Work out the finished part from the listing and answer in its coordinate system (mm). A direction names the side the tool comes from. Coordinates: 2 decimals unless noted, no trailing zeros. Order: outer loops, then holes, each group sorted by start corner. A loop starts at its lowest first (then second) coordinate and runs counter-clockwise, first axis right, second up. Notation, with made-up numbers: M -31,47 L 17,47 A30 ccw 17,81 Z; hole C 75,-9.5 d6. An arc over 180 degrees is marked long. Answer in a Markdown table with one row per item. Add a question column.
Item 1: The part is cut by section C-C (x = -29.5). Write down the section's boundary in (y, z), then the cut area to 3 significant figures.
Item 2: Which of the six approach directions +Z, -Z, +X, -X, +Y, -Y give full straight-line access (tool end or side, diameter ignored) to faces 4 (the face through (63.945, -1, 10)), 5 (the face through (39, -26, 2.67))?
Item 3: The mould has two halves that part along Y. Classify faces 1 (the face through (-1, 1, 20.2)), 2 (the face through (13, 0, 2.67)), 3 (the face through (-1, -42.8, 10)): released by +Y, released by -Y, zero draft, split by the parting line, or undercut.
Item 4: The part is cut by section B-B (z = 6.75). State how many separate pieces and enclosed holes the cut face has, then the cut area to 3 significant figures.
Item 5: The part is cut by section D-D (y = -33). Write down the section's boundary in (x, z) (3 decimals).
Item 6: A flat-ended cylindrical pin translates along its axis: pin 1 Ø6.5 at (x, y) = (8.5, 25.5) entering from +Z. Find the tip coordinate at first contact, or state that the pin passes through.
Item 7: The part is cut by section A-A (y = 31.5). Write down the section's boundary in (x, z) (3 decimals).
Item 8: Consider line 1 (X direction, y = 0.5, z = 7.75) (3 decimals); line 2 (X direction, y = -3, z = 15.75) (3 decimals); line 3 (Z direction, x = -38, y = -34). Determine where each line is inside the solid, lowest interval first. Write a range as from..to.
from build123d import *

# Parameters (mm, degrees)
F0_W     = 127.89
F0_H     = 85.6
F1_DEPTH = 20.2
F3_DEPTH = 17.53


with BuildPart() as f1:
    # F0 (on Top) → F1 (new body)
    with BuildSketch(Plane.XY):
        Rectangle(F0_W, F0_H)
    extrude(amount=F1_DEPTH)

    # F2 (on face) → F3 (cut)
    with BuildSketch(Plane.XY.offset(20.2)):
        with BuildLine():
            Line((-39.005, 26.01), (-39.005, 37.065))
            ThreePointArc((-39.005, 37.065), (-46.822065466, 33.827065466), (-50.06, 26.01))
            Line((-50.06, 26.01), (-39.005, 26.01))
        make_face()
        with BuildLine():
            ThreePointArc((-27.95, 26.01), (-31.187934534, 33.827065466), (-39.005, 37.065))
            Line((-39.005, 37.065), (-39.005, 26.01))
            Line((-39.005, 26.01), (-27.95, 26.01))
        make_face()
        with BuildLine():
            Line((-27.95, 26.01), (-39.005, 26.01))
            Line((-39.005, 26.01), (-39.005, 14.955))
            ThreePointArc((-39.005, 14.955), (-31.187934534, 18.192934534), (-27.95, 26.01))
        make_face()
        with BuildLine():
            Line((-39.005, 14.955), (-39.005, 26.01))
            Line((-39.005, 26.01), (-50.06, 26.01))
            ThreePointArc((-50.06, 26.01), (-46.822065466, 18.192934534), (-39.005, 14.955))
        make_face()
        with BuildLine():
            ThreePointArc((-39.005, 11.055), (-46.822065466, 7.817065466), (-50.06, 0))
            Line((-50.06, 0), (-39.005, 0))
            Line((-39.005, 0), (-39.005, 11.055))
        make_face()
        with BuildLine():
            ThreePointArc((-27.95, 0), (-31.187934534, 7.817065466), (-39.005, 11.055))
            Line((-39.005, 11.055), (-39.005, 0))
            Line((-39.005, 0), (-27.95, 0))
        make_face()
        with BuildLine():
            Line((-39.005, 0), (-50.06, 0))
            ThreePointArc((-50.06, 0), (-46.822065466, -7.817065466), (-39.005, -11.055))
            Line((-39.005, -11.055), (-39.005, 0))
        make_face()
        with BuildLine():
            Line((-27.95, 0), (-39.005, 0))
            Line((-39.005, 0), (-39.005, -11.055))
            ThreePointArc((-39.005, -11.055), (-31.187934534, -7.817065466), (-27.95, 0))
        make_face()
        with BuildLine():
            Line((-39.005, -14.955), (-39.005, -26.01))
            Line((-39.005, -26.01), (-27.95, -26.01))
            ThreePointArc((-27.95, -26.01), (-31.187934534, -18.192934534), (-39.005, -14.955))
        make_face()
        with BuildLine():
            ThreePointArc((-39.005, -14.955), (-46.822065466, -18.192934534), (-50.06, -26.01))
            Line((-50.06, -26.01), (-39.005, -26.01))
            Line((-39.005, -26.01), (-39.005, -14.955))
        make_face()
        with BuildLine():
            Line((-39.005, -26.01), (-50.06, -26.01))
            ThreePointArc((-50.06, -26.01), (-46.822065466, -33.827065466), (-39.005, -37.065))
            Line((-39.005, -37.065), (-39.005, -26.01))
        make_face()
        with BuildLine():
            Line((-39.005, -26.01), (-39.005, -37.065))
            ThreePointArc((-39.005, -37.065), (-31.187934534, -33.827065466), (-27.95, -26.01))
            Line((-27.95, -26.01), (-39.005, -26.01))
        make_face()
        with BuildLine():
            ThreePointArc((-24.05, -26.01), (-20.812065466, -33.827065466), (-12.995, -37.065))
            Line((-12.995, -37.065), (-12.995, -26.01))
            Line((-12.995, -26.01), (-24.05, -26.01))
        make_face()
        with BuildLine():
            Line((-12.995, -26.01), (-12.995, -37.065))
            ThreePointArc((-12.995, -37.065), (-5.177934534, -33.827065466), (-1.94, -26.01))
            Line((-1.94, -26.01), (-12.995, -26.01))
        make_face()
        with BuildLine():
            Line((-12.995, -14.955), (-12.995, -26.01))
            Line((-12.995, -26.01), (-1.94, -26.01))
            ThreePointArc((-1.94, -26.01), (-5.177934534, -18.192934534), (-12.995, -14.955))
        make_face()
        with BuildLine():
            Line((-24.05, -26.01), (-12.995, -26.01))
            Line((-12.995, -26.01), (-12.995, -14.955))
            ThreePointArc((-12.995, -14.955), (-20.812065466, -18.192934534), (-24.05, -26.01))
        make_face()
        with BuildLine():
            Line((-12.995, -11.055), (-12.995, 0))
            Line((-12.995, 0), (-24.05, 0))
            ThreePointArc((-24.05, 0), (-20.812065466, -7.817065466), (-12.995, -11.055))
        make_face()
        with BuildLine():
            Line((-1.94, 0), (-12.995, 0))
            Line((-12.995, 0), (-12.995, -11.055))
            ThreePointArc((-12.995, -11.055), (-5.177934534, -7.817065466), (-1.94, 0))
        make_face()
        with BuildLine():
            ThreePointArc((-1.94, 0), (-5.177934534, 7.817065466), (-12.995, 11.055))
            Line((-12.995, 11.055), (-12.995, 0))
            Line((-12.995, 0), (-1.94, 0))
        make_face()
        with BuildLine():
            Line((-12.995, 0), (-12.995, 11.055))
            ThreePointArc((-12.995, 11.055), (-20.812065466, 7.817065466), (-24.05, 0))
            Line((-24.05, 0), (-12.995, 0))
        make_face()
        with BuildLine():
            Line((-12.995, 14.955), (-12.995, 26.01))
            Line((-12.995, 26.01), (-24.05, 26.01))
            ThreePointArc((-24.05, 26.01), (-20.812065466, 18.192934534), (-12.995, 14.955))
        make_face()
        with BuildLine():
            Line((-1.94, 26.01), (-12.995, 26.01))
            Line((-12.995, 26.01), (-12.995, 14.955))
            ThreePointArc((-12.995, 14.955), (-5.177934534, 18.192934534), (-1.94, 26.01))
        make_face()
        with BuildLine():
            ThreePointArc((-1.94, 26.01), (-5.177934534, 33.827065466), (-12.995, 37.065))
            Line((-12.995, 37.065), (-12.995, 26.01))
            Line((-12.995, 26.01), (-1.94, 26.01))
        make_face()
        with BuildLine():
            Line((-12.995, 26.01), (-12.995, 37.065))
            ThreePointArc((-12.995, 37.065), (-20.812065466, 33.827065466), (-24.05, 26.01))
            Line((-24.05, 26.01), (-12.995, 26.01))
        make_face()
        with BuildLine():
            Line((13.015, 26.01), (13.015, 37.065))
            ThreePointArc((13.015, 37.065), (5.197934534, 33.827065466), (1.96, 26.01))
            Line((1.96, 26.01), (13.015, 26.01))
        make_face()
        with BuildLine():
            ThreePointArc((24.07, 26.01), (20.832065466, 33.827065466), (13.015, 37.065))
            Line((13.015, 37.065), (13.015, 26.01))
            Line((13.015, 26.01), (24.07, 26.01))
        make_face()
        with BuildLine():
            Line((24.07, 26.01), (13.015, 26.01))
            Line((13.015, 26.01), (13.015, 14.955))
            ThreePointArc((13.015, 14.955), (20.832065466, 18.192934534), (24.07, 26.01))
        make_face()
        with BuildLine():
            Line((13.015, 14.955), (13.015, 26.01))
            Line((13.015, 26.01), (1.96, 26.01))
            ThreePointArc((1.96, 26.01), (5.197934534, 18.192934534), (13.015, 14.955))
        make_face()
        with BuildLine():
            Line((13.015, 0), (13.015, 11.055))
            ThreePointArc((13.015, 11.055), (5.197934534, 7.817065466), (1.96, 0))
            Line((1.96, 0), (13.015, 0))
        make_face()
        with BuildLine():
            ThreePointArc((24.07, 0), (20.832065466, 7.817065466), (13.015, 11.055))
            Line((13.015, 11.055), (13.015, 0))
            Line((13.015, 0), (24.07, 0))
        make_face()
        with BuildLine():
            Line((13.015, -11.055), (13.015, 0))
            Line((13.015, 0), (1.96, 0))
            ThreePointArc((1.96, 0), (5.197934534, -7.817065466), (13.015, -11.055))
        make_face()
        with BuildLine():
            ThreePointArc((13.015, -11.055), (20.832065466, -7.817065466), (24.07, 0))
            Line((24.07, 0), (13.015, 0))
            Line((13.015, 0), (13.015, -11.055))
        make_face()
        with BuildLine():
            Line((39.025, -11.055), (39.025, 0))
            Line((39.025, 0), (27.97, 0))
            ThreePointArc((27.97, 0), (31.207934534, -7.817065466), (39.025, -11.055))
        make_face()
        with BuildLine():
            ThreePointArc((39.025, -11.055), (46.842065466, -7.817065466), (50.08, 0))
            Line((50.08, 0), (39.025, 0))
            Line((39.025, 0), (39.025, -11.055))
        make_face()
        with BuildLine():
            Line((39.025, 0), (50.08, 0))
            ThreePointArc((50.08, 0), (46.842065466, 7.817065466), (39.025, 11.055))
            Line((39.025, 11.055), (39.025, 0))
        make_face()
        with BuildLine():
            Line((27.97, 0), (39.025, 0))
            Line((39.025, 0), (39.025, 11.055))
            ThreePointArc((39.025, 11.055), (31.207934534, 7.817065466), (27.97, 0))
        make_face()
        with BuildLine():
            Line((39.025, 14.955), (39.025, 26.01))
            Line((39.025, 26.01), (27.97, 26.01))
            ThreePointArc((27.97, 26.01), (31.207934534, 18.192934534), (39.025, 14.955))
        make_face()
        with BuildLine():
            ThreePointArc((39.025, 14.955), (46.842065466, 18.192934534), (50.08, 26.01))
            Line((50.08, 26.01), (39.025, 26.01))
            Line((39.025, 26.01), (39.025, 14.955))
        make_face()
        with BuildLine():
            ThreePointArc((50.08, 26.01), (46.842065466, 33.827065466), (39.025, 37.065))
            Line((39.025, 37.065), (39.025, 26.01))
            Line((39.025, 26.01), (50.08, 26.01))
        make_face()
        with BuildLine():
            Line((39.025, 26.01), (39.025, 37.065))
            ThreePointArc((39.025, 37.065), (31.207934534, 33.827065466), (27.97, 26.01))
            Line((27.97, 26.01), (39.025, 26.01))
        make_face()
        with BuildLine():
            Line((13.015, -26.01), (24.07, -26.01))
            ThreePointArc((24.07, -26.01), (20.832065466, -18.192934534), (13.015, -14.955))
            Line((13.015, -14.955), (13.015, -26.01))
        make_face()
        with BuildLine():
            Line((1.96, -26.01), (13.015, -26.01))
            Line((13.015, -26.01), (13.015, -14.955))
            ThreePointArc((13.015, -14.955), (5.197934534, -18.192934534), (1.96, -26.01))
        make_face()
        with BuildLine():
            ThreePointArc((1.96, -26.01), (5.197934534, -33.827065466), (13.015, -37.065))
            Line((13.015, -37.065), (13.015, -26.01))
            Line((13.015, -26.01), (1.96, -26.01))
        make_face()
        with BuildLine():
            Line((13.015, -26.01), (13.015, -37.065))
            ThreePointArc((13.015, -37.065), (20.832065466, -33.827065466), (24.07, -26.01))
            Line((24.07, -26.01), (13.015, -26.01))
        make_face()
        with BuildLine():
            Line((27.97, -26.01), (39.025, -26.01))
            Line((39.025, -26.01), (39.025, -14.955))
            ThreePointArc((39.025, -14.955), (31.207934534, -18.192934534), (27.97, -26.01))
        make_face()
        with BuildLine():
            Line((39.025, -26.01), (50.08, -26.01))
            ThreePointArc((50.08, -26.01), (46.842065466, -18.192934534), (39.025, -14.955))
            Line((39.025, -14.955), (39.025, -26.01))
        make_face()
        with BuildLine():
            ThreePointArc((39.025, -37.065), (46.842065466, -33.827065466), (50.08, -26.01))
            Line((50.08, -26.01), (39.025, -26.01))
            Line((39.025, -26.01), (39.025, -37.065))
        make_face()
        with BuildLine():
            Line((39.025, -37.065), (39.025, -26.01))
            Line((39.025, -26.01), (27.97, -26.01))
            ThreePointArc((27.97, -26.01), (31.207934534, -33.827065466), (39.025, -37.065))
        make_face()
    extrude(amount=-F3_DEPTH, mode=Mode.SUBTRACT)


solid = f1.part
Reply:
| question | item | result |
|---|---|---|
| 1 | outline | M -42.8,0 L 42.8,0 L 42.8,20.2 L 31.66,20.2 L 31.66,2.67 L 20.36,2.67 L 20.36,20.2 L 5.65,20.2 L 5.65,2.67 L -5.65,2.67 L -5.65,20.2 L -20.36,20.2 L -20.36,2.67 L -31.66,2.67 L -31.66,20.2 L -42.8,20.2 Z |
| 1 | area | 1,140 mm2 |
| 2 | face 4 | +Z, -Z, +X, +Y, -Y |
| 2 | face 5 | +Z |
| 3 | face 1 | zero draft |
| 3 | face 2 | undercut |
| 3 | face 3 | released by -Y |
| 4 | separate pieces | 1 |
| 4 | enclosed holes | 12 |
| 4 | area | 6,340 mm2 |
| 5 | outline | M -63.945,0 L 63.945,0 L 63.945,20.2 L 47.59,20.2 L 47.59,2.67 L 30.46,2.67 L 30.46,20.2 L 21.58,20.2 L 21.58,2.67 L 4.45,2.67 L 4.45,20.2 L -4.43,20.2 L -4.43,2.67 L -21.56,2.67 L -21.56,20.2 L -30.44,20.2 L -30.44,2.67 L -47.57,2.67 L -47.57,20.2 L -63.945,20.2 Z |
| 6 | pin 1 | stops at z = 2.67 |
| 7 | outline | M -63.945,0 L 63.945,0 L 63.945,20.2 L 48.62,20.2 L 48.62,2.67 L 29.43,2.67 L 29.43,20.2 L 22.61,20.2 L 22.61,2.67 L 3.42,2.67 L 3.42,20.2 L -3.4,20.2 L -3.4,2.67 L -22.59,2.67 L -22.59,20.2 L -29.41,20.2 L -29.41,2.67 L -48.6,2.67 L -48.6,20.2 L -63.945,20.2 Z |
| 8 | line 1 | x = -63.945..-50.049, -27.961..-24.039, -1.951..1.971, 24.059..27.981, 50.069..63.945 |
| 8 | line 2 | x = -63.945..-49.645, -28.365..-23.635, -2.355..2.375, 23.655..28.385, 49.665..63.945 |
| 8 | line 3 | z = 0..2.67 |
